Build history of the part. All positions in model axes, mm. A direction names the side the tool comes from. Give positions to 0.01 mm unless a question says otherwise; leave off trailing zeros. Loops run counter-clockwise (first coordinate to the right, second up) from the corner with the lowest first, then second, coordinate; pieces in that order, holes last. Notation, with made-up numbers: (4, -34.5) - (10, -34.5) arc R28 cw to (10, -4.5) - close; hole circle Ø7 at (65, 49.5). An arc over 180 degrees is marked (long way). Return JSON: item names as keys, results as strings. Group by question number.
1) Slice it at C-C (z = 35). List the corners of the cut face in (x, y), and give its area (3 significant figures).
2) Drop flat-ended pins along their axis: pin 1 (8 mm diameter, centred on y = 9, z = 35, fed in from -X); pin 2 (3.5 mm diameter, centred on x = 7.5, z = 7.5, fed in from +Y); pin 3 (4.5 mm diameter, centred on x = 10.5, y = 5, fed in from -Z); pin 4 (5 mm diameter, centred on x = 5, y = 11, fed in from +Z). Give the stop position or say it passes through.
3) 3-axis set-ups, long thin cutter, end or side, ignore diameter. For faces 1 (the face through (8, 8, 22)), 2 (the face through (12.04, 8.04, 32.69)), 3 (the face through (15, 15, 35)), 4 (the face through (4, 13, 45.5)), 5 (the face through (8, 8, 48)): which of +Z, -Z, +X, -X, +Y, -Y reach the whole face in a straight line?
4) Slice it at B-B (y = 21.25). List the corners of the cut face in (x, z), and give its area (3 significant figures).
5) Slice it at A-A (x = 4). List the corners of the cut face in (y, z).
6) Mould opens along X. For faces 6 (the face through (6.906, 21.521, 8.932)), 7 (the face through (0, 18, 55)), 8 (the face through (11, 25, 35)) say: released by +X, released by -X, zero draft, split by the parting line, or undercut.
7) Slice it at D-D (x = 9.75). List the corners of the cut face in (y, z), and give its area (3 significant figures).
8) Drill centre lines: probe 1 along Z at (x, y) = (2.25, 2.5); probe 2 along Z at (x, y) = (7.5, 22); probe 3 along Y at (x, z) = (12.45, 35). Where is each one in solid material? Low to high. Write a range as from..to.
```python
from build123d import *

# Parameters (mm, degrees)
SKETCH_1_W          = 15
SKETCH_1_H          = 70
EXTRUDE_1_DEPTH     = 25
CUT_EXTRUDE_1_DEPTH = 40
SKETCH_3_W          = 9
SKETCH_3_H          = 21
CUT_EXTRUDE_2_DEPTH = 76.828754441
SKETCH_5_R          = 1.55
CUT_EXTRUDE_3_DEPTH = 76.828754441
SKETCH_6_R          = 2.5
CUT_EXTRUDE_4_DEPTH = 76.828754441


with BuildPart() as part:
    # 草图1 → 凸台-拉伸1 (new body)
    with BuildSketch(Plane(origin=(0, 0, 0), x_dir=(1, 0, 0), z_dir=(0, 1, 0))):
        with Locations((7.5, -35)):
            Rectangle(SKETCH_1_W, SKETCH_1_H)
    extrude(amount=EXTRUDE_1_DEPTH)

    # 草图2 → 切除-拉伸1 (cut)
    with BuildSketch(Plane(origin=(15, 0, 0), x_dir=(0, 0, -1), z_dir=(1, 0, 0))):
        Polygon((-70, 20), (-48, 15), (-48, 0), (-70, 0), align=None)
        Polygon((0, 20), (-22, 15), (-22, 0), (0, 0), align=None)
    extrude(amount=-CUT_EXTRUDE_1_DEPTH, mode=Mode.SUBTRACT)

    # 草图3 → 切除-拉伸2 (cut, through all)
    with BuildSketch(Plane(origin=(0, 25, 0), x_dir=(1, 0, 0), z_dir=(0, 1, 0))):
        with Locations((4.5, -35)):
            Rectangle(SKETCH_3_W, SKETCH_3_H)
    extrude(amount=-CUT_EXTRUDE_2_DEPTH, mode=Mode.SUBTRACT)

    # 草图5 → 切除-拉伸3 (cut, through all)
    with BuildSketch(Plane(origin=(0, 25, 0), x_dir=(1, 0, 0), z_dir=(0, 1, 0))):
        with Locations(Location((7.5, -7.5, 0), (0, 0, 270))):
            Circle(SKETCH_5_R)
        with Locations(Location((7.5, -62.5, 0), (0, 0, 270))):
            Circle(SKETCH_5_R)
    extrude(amount=-CUT_EXTRUDE_3_DEPTH, mode=Mode.SUBTRACT)

    # 草图6 → 切除-拉伸4 (cut, through all)
    with BuildSketch(Plane(origin=(15, 0, 0), x_dir=(0, 0, -1), z_dir=(1, 0, 0))):
        with Locations((-35, 9)):
            Circle(SKETCH_6_R)
    extrude(amount=-CUT_EXTRUDE_4_DEPTH, mode=Mode.SUBTRACT)


solid = part.part
```
Results:
{
 "1": {"outline": "(9, 0) - (15, 0) - (15, 6.5) - (9, 6.5) - close; (9, 11.5) - (15, 11.5) - (15, 25) - (9, 25) - close", "area": "120 mm2"},
 "2": {"pin 1": "x = 9", "pin 2": "y = 25", "pin 3": "z = 22", "pin 4": "z = 48"},
 "3": {"face 1": "-Z, +X, -X, -Y", "face 2": "+X, -X", "face 3": "+Z, -Z, +X, +Y, -Y", "face 4": "-X, +Y, -Y", "face 5": "+Z, +X, -X, -Y"},
 "4": {"outline": "(0, 0) - (15, 0) - (15, 70) - (0, 70) - (0, 45.5) - (9, 45.5) - (9, 24.5) - (0, 24.5) - close; hole circle Ø3.1 at (7.5, 7.5); hole circle Ø3.1 at (7.5, 62.5)", "area": "846 mm2"},
 "5": {"outline": "(0, 22) - (15, 22) - (20, 0) - (25, 0) - (25, 24.5) - (0, 24.5) - close; (0, 45.5) - (25, 45.5) - (25, 70) - (20, 70) - (15, 48) - (0, 48) - close"},
 "6": {"face 6": "undercut", "face 7": "released by -X", "face 8": "zero draft"},
 "7": {"outline": "(0, 22) - (15, 22) - (20, 0) - (25, 0) - (25, 70) - (20, 70) - (15, 48) - (0, 48) - close; hole circle Ø5 at (9, 35)", "area": "960 mm2"},
 "8": {"probe 1": "22..24.5, 45.5..48", "probe 2": "0..5.95, 9.05..24.5, 45.5..60.95, 64.05..70", "probe 3": "0..6.5, 11.5..25"}
}
